Input: part model. Units: mm. Frame: model coordinates. A direction names the side the tool comes from. Round coordinates to 2 decimals unless told otherwise and drop trailing zeros. Loops run counter-clockwise (first coordinate to the right, second up) from the corner with the lowest first, then second, coordinate; pieces in that order, holes last.
(1) Cut plane B-B, the plane z = -9. Output: boundary loops of the cut face in (x, y), and give its area (3 significant figures).
(2) Cut plane D-D, the plane y = 24.5. Output: boundary loops of the cut face in (x, z).
(3) Draft query along Y for faces 1 (the face through (1.15, 0.66, -10.14)), 2 (the face through (72.916, 38.096, 1.964)), 3 (the face through (-0.4, 45.5, 25)). Return one class per face: released by +Y, released by -Y, zero draft, split by the parting line, or undercut.
(4) Access query for faces 4 (the face through (-66.547, 36.621, -17.288)), 5 (the face through (76.69, 39.67, 2.21)). Directions: +Z, -Z, +X, -X, +Y, -Y. A direction counts if a zero-diameter tool reaches every point of the face in a straight line with its end or side. Return the directions, or none.
(5) Cut plane C-C, the plane x = -35.5. Output: boundary loops of the cut face in (y, z), and give its area (3 significant figures).
(6) Line query: line 1 (X direction, y = 41, z = -5); line 2 (Y direction, x = 76, z = 11); line 3 (Y direction, x = -34, z = 20). Output: solid intervals per line, ascending.
(7) Cut plane A-A, the plane z = 15.5. Output: boundary loops of the cut face in (x, y).
(8) First-contact query: pin 1 Ø0.9 at (y, z) = (46, -11.5) entering from -X; pin 2 Ø5 at (x, y) = (54.5, 19.5) entering from -Z; pin 3 Ø3.5 at (x, y) = (76, -41) entering from +Z. Flat tips, straight axial feed; report the tip coordinate or a pass-through.
from build123d import *

# Parameters (mm, degrees)
SKIZZE1_W                       = 164
SKIZZE1_H                       = 94
AUFSATZ_LINEAR_AUSTRAGEN1_DEPTH = 25
AUFSATZ_LINEAR_AUSTRAGEN2_DEPTH = 164
SCHNITT_LINEAR_AUSTRAGEN1_REACH = 106.68
AUFSATZ_LINEAR_AUSTRAGEN3_REACH = 106.68
SKIZZE4_R                       = 4.236153916
SKIZZE4_R_2                     = 1.5
SCHNITT_LINEAR_AUSTRAGEN2_DEPTH = 4.05
VERRUNDUNG1_R                   = 5
SKIZZE7_W                       = 9
SKIZZE7_H                       = 4
SCHNITT_LINEAR_AUSTRAGEN4_DEPTH = 4.05
SKIZZE8_R                       = 5.5
SCHNITT_LINEAR_AUSTRAGEN5_DEPTH = 1


with BuildPart() as part:
    # Skizze1 → Aufsatz-Linear austragen1 (new body)
    with BuildSketch(Plane.XY):
        Rectangle(SKIZZE1_W, SKIZZE1_H)
    extrude(amount=AUFSATZ_LINEAR_AUSTRAGEN1_DEPTH)

    # Skizze2 → Aufsatz-Linear austragen2 (add)
    with BuildSketch(Plane(origin=(82, 0, 0), x_dir=(0, 0, -1), z_dir=(1, 0, 0))):
        Polygon((0, -47), (0, 47), (20, 47), align=None)
    extrude(amount=-AUFSATZ_LINEAR_AUSTRAGEN2_DEPTH)

    # Schnitt-Linear austragen1: up to this plane
    schnitt_linear_austragen1_end = Plane(origin=(-82, 47.416215289, -18.043788142), z_dir=(0, -0.20810764446485866, -0.9781059289848355))
    # Skizze3 → Schnitt-Linear austragen1 (cut, up to the surface)
    with BuildSketch(Plane.XY.offset(25), mode=Mode.PRIVATE) as schnitt_linear_austragen1_sk1:
        with BuildLine():
            Line((-75.15, -45.15), (75.15, -45.15))
            ThreePointArc((75.15, -45.15), (78.685533906, -43.685533906), (80.15, -40.15))
            Line((80.15, -40.15), (80.15, 40.15))
            ThreePointArc((80.15, 40.15), (78.685533906, 43.685533906), (75.15, 45.15))
            Line((75.15, 45.15), (-75.15, 45.15))
            ThreePointArc((-75.15, 45.15), (-78.685533906, 43.685533906), (-80.15, 40.15))
            Line((-80.15, 40.15), (-80.15, -40.15))
            ThreePointArc((-80.15, -40.15), (-78.685533906, -43.685533906), (-75.15, -45.15))
        make_face()
    schnitt_linear_austragen1_tool1 = split(extrude(schnitt_linear_austragen1_sk1.sketch, amount=-SCHNITT_LINEAR_AUSTRAGEN1_REACH, mode=Mode.PRIVATE), bisect_by=schnitt_linear_austragen1_end, keep=Keep.BOTH, mode=Mode.PRIVATE)
    add(schnitt_linear_austragen1_tool1.solids().sort_by_distance((0, 0, 25))[0], mode=Mode.SUBTRACT)

    # Aufsatz-Linear austragen3: up to this plane
    aufsatz_linear_austragen3_end = Plane(origin=(-82, 47.416215289, -18.043788142), z_dir=(0, -0.20810764446485866, -0.9781059289848355))
    # Skizze4 → Aufsatz-Linear austragen3 (add, up to the surface)
    with BuildSketch(Plane.XY.offset(25), mode=Mode.PRIVATE) as aufsatz_linear_austragen3_sk1:
        with Locations((-76, 41)):
            Circle(SKIZZE4_R)
        with Locations((-76, 41)):
            Circle(SKIZZE4_R_2, mode=Mode.SUBTRACT)
    aufsatz_linear_austragen3_tool1 = split(extrude(aufsatz_linear_austragen3_sk1.sketch, amount=-AUFSATZ_LINEAR_AUSTRAGEN3_REACH, mode=Mode.PRIVATE), bisect_by=aufsatz_linear_austragen3_end, keep=Keep.BOTH, mode=Mode.PRIVATE)
    add(aufsatz_linear_austragen3_tool1.solids().sort_by_distance((-80.116337, 41, 25))[0])
    # Skizze4 → Aufsatz-Linear austragen3 (add, up to the surface)
    with BuildSketch(Plane.XY.offset(25), mode=Mode.PRIVATE) as aufsatz_linear_austragen3_sk2:
        with Locations((-76, -41)):
            Circle(SKIZZE4_R)
        with Locations((-76, -41)):
            Circle(SKIZZE4_R_2, mode=Mode.SUBTRACT)
    aufsatz_linear_austragen3_tool2 = split(extrude(aufsatz_linear_austragen3_sk2.sketch, amount=-AUFSATZ_LINEAR_AUSTRAGEN3_REACH, mode=Mode.PRIVATE), bisect_by=aufsatz_linear_austragen3_end, keep=Keep.BOTH, mode=Mode.PRIVATE)
    add(aufsatz_linear_austragen3_tool2.solids().sort_by_distance((-80.116337, -41, 25))[0])
    # Skizze4 → Aufsatz-Linear austragen3 (add, up to the surface)
    with BuildSketch(Plane.XY.offset(25), mode=Mode.PRIVATE) as aufsatz_linear_austragen3_sk3:
        with Locations((76, -41)):
            Circle(SKIZZE4_R)
        with Locations((76, -41)):
            Circle(SKIZZE4_R_2, mode=Mode.SUBTRACT)
    aufsatz_linear_austragen3_tool3 = split(extrude(aufsatz_linear_austragen3_sk3.sketch, amount=-AUFSATZ_LINEAR_AUSTRAGEN3_REACH, mode=Mode.PRIVATE), bisect_by=aufsatz_linear_austragen3_end, keep=Keep.BOTH, mode=Mode.PRIVATE)
    add(aufsatz_linear_austragen3_tool3.solids().sort_by_distance((71.883663, -41, 25))[0])
    # Skizze4 → Aufsatz-Linear austragen3 (add, up to the surface)
    with BuildSketch(Plane.XY.offset(25), mode=Mode.PRIVATE) as aufsatz_linear_austragen3_sk4:
        with Locations((76, 41)):
            Circle(SKIZZE4_R)
        with Locations((76, 41)):
            Circle(SKIZZE4_R_2, mode=Mode.SUBTRACT)
    aufsatz_linear_austragen3_tool4 = split(extrude(aufsatz_linear_austragen3_sk4.sketch, amount=-AUFSATZ_LINEAR_AUSTRAGEN3_REACH, mode=Mode.PRIVATE), bisect_by=aufsatz_linear_austragen3_end, keep=Keep.BOTH, mode=Mode.PRIVATE)
    add(aufsatz_linear_austragen3_tool4.solids().sort_by_distance((71.883663, 41, 25))[0])

    # Skizze6 → Schnitt-Linear austragen2 (cut)
    with BuildSketch(Plane.XY.offset(25)):
        with BuildLine():
            Line((-75.15, -45.15), (75.15, -45.15))
            ThreePointArc((75.15, -45.15), (78.685533906, -43.685533906), (80.15, -40.15))
            Line((80.15, -40.15), (80.15, 40.15))
            ThreePointArc((80.15, 40.15), (78.685533906, 43.685533906), (75.15, 45.15))
            Line((75.15, 45.15), (-75.15, 45.15))
            ThreePointArc((-75.15, 45.15), (-78.685533906, 43.685533906), (-80.15, 40.15))
            Line((-80.15, 40.15), (-80.15, -40.15))
            ThreePointArc((-80.15, -40.15), (-78.685533906, -43.685533906), (-75.15, -45.15))
        make_face()
    extrude(amount=-SCHNITT_LINEAR_AUSTRAGEN2_DEPTH, mode=Mode.SUBTRACT)

    # Verrundung1
    verrundung1_edges = [part.edges().sort_by_distance(p)[0] for p in [
        (82, -47, 12.5),
        (-82, -47, 12.5),
        (-82, 47, 2.5),
        (82, 47, 2.5),
    ]]
    fillet(verrundung1_edges, radius=VERRUNDUNG1_R)

    # Skizze7 → Schnitt-Linear austragen4 (cut)
    with BuildSketch(Plane(origin=(0, 47, 0), x_dir=(1, 0, 0), z_dir=(0, 1, 0))):
        with Locations((13.5, 12.561614676)):
            Rectangle(SKIZZE7_W, SKIZZE7_H)
    extrude(amount=-SCHNITT_LINEAR_AUSTRAGEN4_DEPTH, mode=Mode.SUBTRACT)

    # Skizze8 → Schnitt-Linear austragen5 (cut)
    with BuildSketch(Plane(origin=(0, -2.035513209, -9.566912083), x_dir=(-1, 0, 0), z_dir=(0, -0.20810764446485866, -0.9781059289848355))):
        with Locations(Location((-72, 40.133131552, 0), (0, 0, 90))):
            Circle(SKIZZE8_R)
        with Locations(Location((72, 40.133131552, 0), (0, 0, 90))):
            Circle(SKIZZE8_R)
        with Locations(Location((72, -35.970978662, 0), (0, 0, 90))):
            Circle(SKIZZE8_R)
        with Locations(Location((-72, -35.970978662, 0), (0, 0, 90))):
            Circle(SKIZZE8_R)
    extrude(amount=-SCHNITT_LINEAR_AUSTRAGEN5_DEPTH, mode=Mode.SUBTRACT)


solid = part.part
Reported:
1. outline: (-82, -4.7) - (82, -4.7) - (82, 42) arc R5 ccw to (77, 47) - (-77, 47) arc R5 ccw to (-82, 42) - close; hole (-80.15, 4.91) - (80.15, 4.91) - (80.15, 40.15) arc R4.24 cw (long way) to (75.15, 45.15) - (-75.15, 45.15) arc R4.24 cw (long way) to (-80.15, 40.15) - close; hole circle Ø3 at (-76, 41); hole circle Ø3 at (76, 41)
1. area: 2,120 mm2
2. outline: (-82, -15.21) - (82, -15.21) - (82, 25) - (80.15, 25) - (80.15, -13.17) - (-80.15, -13.17) - (-80.15, 25) - (-82, 25) - close
3. face 1: released by -Y
3. face 2: undercut
3. face 3: zero draft
4. face 4: none
4. face 5: +Z
5. outline: (-47, 0) - (47, -20) - (47, 25) - (45.15, 25) - (45.15, -17.56) - (-45.15, 1.65) - (-45.15, 25) - (-47, 25) - close
5. area: 314 mm2
6. line 1: x = -82 to -77.5, -74.5 to -71.76, 71.76 to 74.5, 77.5 to 82
6. line 2: y = -47 to -42.5, -39.5 to -36.76, 36.76 to 39.5, 42.5 to 47
6. line 3: y = -47 to -45.15, 45.15 to 47
7. outline: (-82, -42) arc R5 ccw to (-77, -47) - (77, -47) arc R5 ccw to (82, -42) - (82, 42) arc R5 ccw to (77, 47) - (-77, 47) arc R5 ccw to (-82, 42) - close; hole (-80.15, -40.15) arc R4.24 cw (long way) to (-75.15, -45.15) - (75.15, -45.15) arc R4.24 cw (long way) to (80.15, -40.15) - (80.15, 40.15) arc R4.24 cw (long way) to (75.15, 45.15) - (-75.15, 45.15) arc R4.24 cw (long way) to (-80.15, 40.15) - close; hole circle Ø3 at (-76, -41); hole circle Ø3 at (-76, 41); hole circle Ø3 at (76, -41); hole circle Ø3 at (76, 41)
8. pin 1: stops at x = -80.52
8. pin 2: stops at z = -14.68
8. pin 3: stops at z = 20.95
